Here's the drawing with two shaded views (mm, measured from the low corner). I have some questions. A direction names the side the tool comes from. Round coordinates to 2 decimals unless told otherwise and drop trailing zeros. Order: outer loops, then holes, each group sorted by start corner. A loop starts at its lowest first (then second) coordinate and runs counter-clockwise, first axis right, second up. Notation, with made-up numbers: (-0.5, 16) -> (24.5, 16) arc R27 cw to (24.5, 48) -> close; hole circle Ø3 at (53.5, 31). An arc over 180 degrees is marked (long way). One line per question, with ' | ' between items.
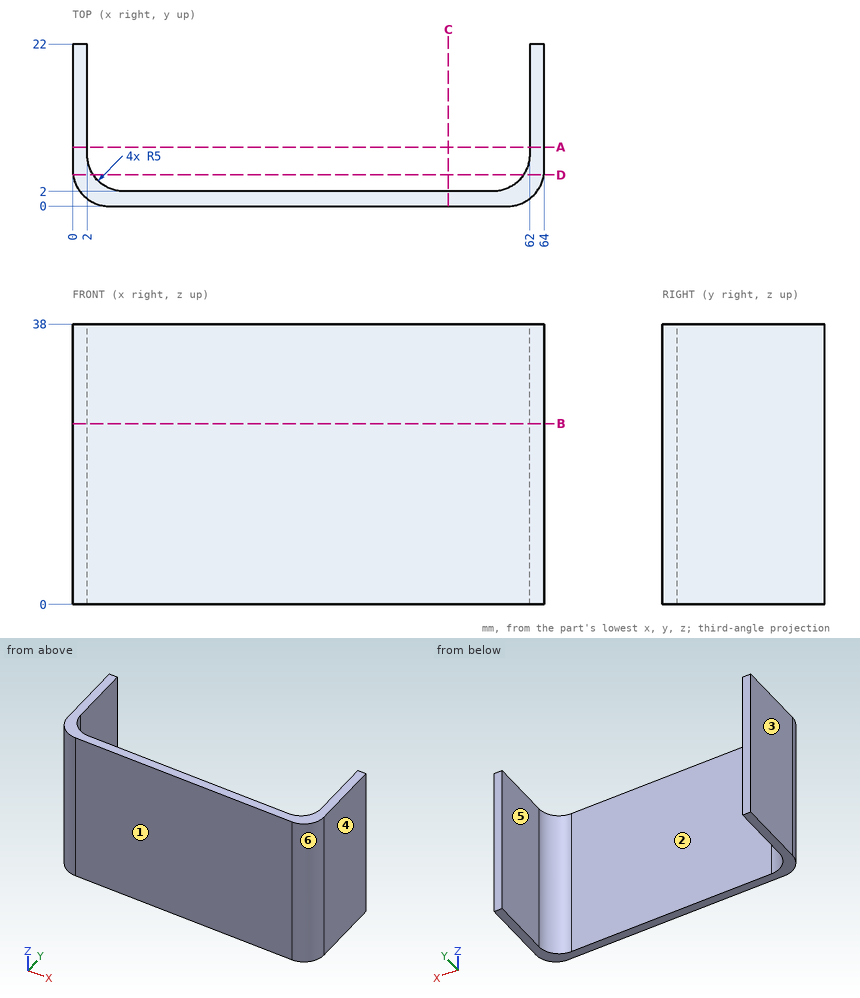
1. I want a section at A-A on y = 8. List the corners of the cut face in (x, z) for me.
From the geometry:
outline: (0, 0) -> (2, 0) -> (2, 38) -> (0, 38) -> close; (62, 0) -> (64, 0) -> (64, 38) -> (62, 38) -> close
2. I want a section at C-C on x = 51. List the corners of the cut face in (y, z) for me.
From the geometry:
outline: (0, 0) -> (2, 0) -> (2, 38) -> (0, 38) -> close
3. On a 3-axis mill with a long thin cutter (end or side, diameter ignored), from which of +Z, -Z, +X, -X, +Y, -Y can I reach the whole of each face in a straight line? I mean the marked faces 5 and 6. Say none if no direction works.
From the geometry:
face 5: +Z, -Z, +Y | face 6: +Z, -Z, +X, -Y
4. I want a section at B-B on z = 24.5. List the corners of the cut face in (x, y) for me.
From the geometry:
outline: (0, 5) arc R5 ccw to (5, 0) -> (59, 0) arc R5 ccw to (64, 5) -> (64, 22) -> (62, 22) -> (62, 7) arc R5 cw to (57, 2) -> (7, 2) arc R5 cw to (2, 7) -> (2, 22) -> (0, 22) -> close
5. I need wall thicknesses on probe 1 along X at (y, z) = (12, 28); probe 2 along Y at (x, z) = (10, 14); probe 3 along X at (y, z) = (4.75, 16.5). Which ranges of each line are inside material? Lowest first, please.
From the geometry:
probe 1: x = 0 to 2, 62 to 64 | probe 2: y = 0 to 2 | probe 3: x = 0.01 to 2.53, 61.47 to 63.99
6. I want a section at D-D on y = 4.25. List the corners of the cut face in (x, z) for me.
From the geometry:
outline: (0.06, 0) -> (2.82, 0) -> (2.82, 38) -> (0.06, 38) -> close; (61.18, 0) -> (63.94, 0) -> (63.94, 38) -> (61.18, 38) -> close
7. If we mould it in two halves opening along X, with no side actions, what happens to the marked faces 1, 2, 3 and 4? For each: pulls with the +X half, pulls with the -X half, needs draft (parallel to the pull), parting line crosses it, or undercut.
From the geometry:
face 1: needs draft | face 2: undercut | face 3: pulls with the -X half | face 4: pulls with the +X half
8. I'm going to push flat-ended pins straight in: pin 1 (10 mm diameter, centred on x = 49.5, y = 8.5, fed in from +Z); pin 2 (1.5 mm diameter, centred on x = 50, z = 22, fed in from +Y). Where does each tip first touch, or does it pass through?
From the geometry:
pin 1: passes through | pin 2: stops at y = 2
